Check sheet for the modelled part. Datum: model origin and axes. Units: mm. A direction names the side the tool comes from. Give positions to 0.01 mm unless a question says otherwise; leave off trailing zeros. Write each loop counter-clockwise with the first axis right and the second up, starting at its lowest first coordinate (ties: lowest second). Pieces come first, ordered by that corner, then holes. Notation, with made-up numbers: M 1,78.25 L 41,78.25 A22 cw 41,100.25 Z; hole C -24.75,10 d6. An arc over 180 degrees is marked long. Write item = value, one per line. Start each with the question number.
1) Sectioned sample at D-D, the plane z = 20.5. Record the cut outline in (x, y).
2) Gauge pin test, flat ends, axial feed: pin 1 (3 mm diameter, centred on y = 22.5, z = -29, fed in from -X); pin 2 (12 mm diameter, centred on y = 30, z = -3.5, fed in from -X); pin 3 (3 mm diameter, centred on x = 10, y = 73.5, fed in from +Z); pin 4 (5 mm diameter, centred on x = -9, z = -19, fed in from +Y). Record the tip position at first contact, or that the pin passes through.
3) Sectioned sample at C-C, the plane y = 47. Record the cut outline in (x, z), then the cut area to 3 significant figures.
4) Scan lines: L1, parallel to Z at x = 0, y = 63; L2, parallel to Z at x = 29, y = 57; L3, parallel to Z at x = 32, y = 72. Record each from-to range of solid material in increasing order.
5) Set-up check for faces 1 (the face through (-61.5, 36.9, 0.2)), 2 (the face through (0, 7.6, -63)), 3 (the face through (29, 0, -53)): record each of +Z, -Z, +X, -X, +Y, -Y from which the full face is reachable in a straight line by a thin tool's end or side.
6) Draft check along X on faces 4 (the face through (0, 4, -64.566)), 5 (the face through (-1, 71, -27)). Enter one of: pulls with the +X half, pulls with the -X half, needs draft (parallel to the pull), parting line crosses it, or undercut.
7) Sectioned sample at A-A, the plane z = 0. Record the cut outline in (x, y), then the cut area to 3 significant figures.
8) Sectioned sample at B-B, the plane x = 15. Record the cut outline in (y, z), then the cut area to 3 significant figures.
from build123d import *

# Parameters (mm, degrees)
SKETCH1_R               = 65
SKETCH1_R_2             = 60
BOSS_EXTRUDE1_DEPTH     = 55
SKETCH2_R               = 65
BOSS_EXTRUDE2_DEPTH     = 20
SKETCH3_R               = 4.1
SKETCH3_W               = 45
SKETCH3_H               = 45
CUT_EXTRUDE1_DEPTH      = 76
SKETCH5_W               = 45
SKETCH5_H               = 20
CUT_EXTRUDE2_DEPTH      = 18
SKETCH6_R               = 51
CUT_EXTRUDE3_DEPTH      = 6
SKETCH7_R               = 7
SKETCH7_R_2             = 4.1
BOSS_EXTRUDE3_DEPTH     = 6
SKETCH8_R               = 39
CUT_EXTRUDE4_DEPTH      = 10
CUT_EXTRUDE5_DEPTH      = 1
CUT_EXTRUDE5_DEPTH_BACK = 76
SKETCH10_W              = 15
SKETCH10_H              = 12.8
CUT_EXTRUDE6_DEPTH      = 10
CUT_EXTRUDE7_START      = -3
SKETCH11_W              = 20
SKETCH11_H              = 20
CUT_EXTRUDE7_DEPTH      = 10
SKETCH12_R              = 7.5
CUT_EXTRUDE8_DEPTH      = 6
SKETCH13_R              = 10.5
CUT_EXTRUDE9_DEPTH      = 56
CUT_EXTRUDE9_DEPTH_BACK = 6


with BuildPart() as part:
    # Sketch1 → Boss-Extrude1 (new body)
    with BuildSketch(Plane(origin=(0, 0, 0), x_dir=(1, 0, 0), z_dir=(0, 1, 0))):
        with Locations(Location((0, 0, 0), (0, 0, 270))):  # turned: the seam where the file's is
            Circle(SKETCH1_R)
        with Locations(Location((0, 0, 0), (0, 0, 270))):  # turned: the seam where the file's is
            Circle(SKETCH1_R_2, mode=Mode.SUBTRACT)
    extrude(amount=BOSS_EXTRUDE1_DEPTH)

    # Sketch2 → Boss-Extrude2 (add)
    with BuildSketch(Plane(origin=(0, 55, 0), x_dir=(1, 0, 0), z_dir=(0, 1, 0))):
        with Locations(Location((0, 0, 0), (0, 0, 270))):  # turned: the seam where the file's is
            Circle(SKETCH2_R)
    extrude(amount=BOSS_EXTRUDE2_DEPTH)

    # Sketch3 → Cut-Extrude1 (cut, through all)
    with BuildSketch(Plane(origin=(0, 75, 0), x_dir=(1, 0, 0), z_dir=(0, 1, 0))):
        with Locations(Location((-33.234018716, -33.234018716, 0), (0, 0, 270))):  # turned: the seam where the file's is
            Circle(SKETCH3_R)
        with Locations(Location((-33.234018716, 33.234018716, 0), (0, 0, 270))):  # turned: the seam where the file's is
            Circle(SKETCH3_R)
        with Locations(Location((33.234018716, 33.234018716, 0), (0, 0, 270))):  # turned: the seam where the file's is
            Circle(SKETCH3_R)
        with Locations(Location((33.234018716, -33.234018716, 0), (0, 0, 270))):  # turned: the seam where the file's is
            Circle(SKETCH3_R)
        Rectangle(SKETCH3_W, SKETCH3_H)
    extrude(amount=-CUT_EXTRUDE1_DEPTH, mode=Mode.SUBTRACT)

    # Sketch5 → Cut-Extrude2 (cut)
    with BuildSketch(Plane.XZ.offset(-55)):
        with Locations((0, 32.5)):
            Rectangle(SKETCH5_W, SKETCH5_H)
    extrude(amount=-CUT_EXTRUDE2_DEPTH, mode=Mode.SUBTRACT)

    # Sketch6 → Cut-Extrude3 (cut)
    with BuildSketch(Plane.XZ.offset(-55)):
        Circle(SKETCH6_R)
    extrude(amount=-CUT_EXTRUDE3_DEPTH, mode=Mode.SUBTRACT)

    # Sketch7 → Boss-Extrude3 (add)
    with BuildSketch(Plane.XZ.offset(-61)):
        with Locations((-33.234018716, -33.234018716)):
            Circle(SKETCH7_R)
        with Locations(Location((-33.234018716, -33.234018716, 0), (0, 0, 90))):  # turned: the seam where the file's is
            Circle(SKETCH7_R_2, mode=Mode.SUBTRACT)
        with Locations((-33.234018716, 33.234018716)):
            Circle(SKETCH7_R)
        with Locations(Location((-33.234018716, 33.234018716, 0), (0, 0, 90))):  # turned: the seam where the file's is
            Circle(SKETCH7_R_2, mode=Mode.SUBTRACT)
        with Locations((33.234018716, -33.234018716)):
            Circle(SKETCH7_R)
        with Locations(Location((33.234018716, -33.234018716, 0), (0, 0, 90))):  # turned: the seam where the file's is
            Circle(SKETCH7_R_2, mode=Mode.SUBTRACT)
        with Locations((33.234018716, 33.234018716)):
            Circle(SKETCH7_R)
        with Locations(Location((33.234018716, 33.234018716, 0), (0, 0, 90))):  # turned: the seam where the file's is
            Circle(SKETCH7_R_2, mode=Mode.SUBTRACT)
    extrude(amount=BOSS_EXTRUDE3_DEPTH)

    # Sketch8 → Cut-Extrude4 (cut)
    with BuildSketch(Plane.XZ.offset(-61)):
        Circle(SKETCH8_R)
    extrude(amount=-CUT_EXTRUDE4_DEPTH, mode=Mode.SUBTRACT)

    # Sketch9 → Cut-Extrude5 (cut, two sides)
    with BuildSketch(Plane.XZ) as cut_extrude5_sk:
        Polygon((314.441485957, -64.565857851), (7.5, -64.565857851), (-7.5, -64.565857851), (-314.441485957, -64.565857851), (-314.441485957, -678.448829765), (314.441485957, -678.448829765), align=None)
    extrude(amount=CUT_EXTRUDE5_DEPTH, mode=Mode.SUBTRACT)
    extrude(cut_extrude5_sk.sketch, amount=-CUT_EXTRUDE5_DEPTH_BACK, mode=Mode.SUBTRACT)

    # Sketch10 → Cut-Extrude6 (cut)
    with BuildSketch(Plane(origin=(0, 0, -64.565857851), x_dir=(-1, 0, 0), z_dir=(0, 0, -1))):
        with Locations((0, 14)):
            Rectangle(SKETCH10_W, SKETCH10_H)
    extrude(amount=-CUT_EXTRUDE6_DEPTH, mode=Mode.SUBTRACT)

    # Sketch11 → Cut-Extrude7 (cut)
    with BuildSketch(Plane(origin=(0, 0, -64.565857851), x_dir=(-1, 0, 0), z_dir=(0, 0, -1)).offset(CUT_EXTRUDE7_START)):
        with Locations((0, 14)):
            Rectangle(SKETCH11_W, SKETCH11_H)
    extrude(amount=-CUT_EXTRUDE7_DEPTH, mode=Mode.SUBTRACT)

    # Sketch12 → Cut-Extrude8 (cut)
    with BuildSketch(Plane.XZ.offset(-55)):
        with Locations((0, 51)):
            Circle(SKETCH12_R)
    extrude(amount=-CUT_EXTRUDE8_DEPTH, mode=Mode.SUBTRACT)

    # Sketch13 → Cut-Extrude9 (cut, two sides)
    with BuildSketch(Plane.XZ.offset(-55)) as cut_extrude9_sk:
        with Locations((-51, 0)):
            Circle(SKETCH13_R)
    extrude(amount=CUT_EXTRUDE9_DEPTH, mode=Mode.SUBTRACT)
    extrude(cut_extrude9_sk.sketch, amount=-CUT_EXTRUDE9_DEPTH_BACK, mode=Mode.SUBTRACT)


solid = part.part
Data:
q1.outline = M -61.68,0 L -56.39,0 L -56.39,55 L -46.7,55 L -46.7,61 L -33.18,61 L -33.18,71 L -22.5,71 L -22.5,75 L -61.68,75 Z; M 22.5,71 L 33.18,71 L 33.18,61 L 46.7,61 L 46.7,55 L 56.39,55 L 56.39,0 L 61.68,0 L 61.68,75 L 22.5,75 Z
q2.pin_1 = -58.9
q2.pin_2 = -65
q2.pin_3 = 64.44
q2.pin_4 = through
q3.outline = M -7.5,-64.57 L 7.5,-64.57 A65 ccw long Z; hole M -59.71,-5.86 A60 ccw long -59.71,5.86 A10.5 ccw Z
q3.area = 1,950 mm2
q4.L1 = -64.57 to -39, 42.5 to 65
q4.L2 = -58.17 to -41.95, -38.81 to -27.66, 27.66 to 38.81, 41.95 to 58.17
q4.L3 = -56.58 to -37.14, -29.32 to 29.32, 37.14 to 56.58
q5.face_1 = -Y
q5.face_2 = -Z
q5.face_3 = +Z, -Z, +X, -X, -Y
q6.face_4 = needs draft
q6.face_5 = undercut
q7.outline = M -65,0 L -61.5,0 L -61.5,61 L -39,61 L -39,71 L -22.5,71 L -22.5,75 L -65,75 Z; M 22.5,71 L 39,71 L 39,61 L 51,61 L 51,55 L 60,55 L 60,0 L 65,0 L 65,75 L 22.5,75 Z
q7.area = 1,430 mm2
q8.outline = M 0,-63.25 L 75,-63.25 L 75,-22.5 L 71,-22.5 L 71,-36 L 61,-36 L 61,-48.74 L 55,-48.74 L 55,-58.09 L 0,-58.09 Z; M 0,58.09 L 55,58.09 L 55,48.74 L 61,48.74 L 61,42.5 L 73,42.5 L 73,22.5 L 75,22.5 L 75,63.25 L 0,63.25 Z
q8.area = 1,510 mm2
